Input: part model. Units: mm. Frame: model coordinates. Face numbers are marked on the shaded views. A direction names the side the tool comes from. Round coordinates to 2 decimals unless told otherwise and drop trailing zeros. Loops run counter-clockwise (first coordinate to the right, second up) from the corner with the lowest first, then second, coordinate; pieces in that order, holes last.
1) Access query for the marked faces 1 and 2. Directions: +Z, -Z, +X, -X, +Y, -Y. A direction counts if a zero-diameter tool reaches every point of the face in a straight line with its end or side. Return the directions, or none.
2) Section D-D, the plane z = -15. Return loops of the section in (x, y), and give its area (3 significant figures).
3) Section A-A, the plane y = 37. Return loops of the section in (x, z).
4) Section C-C, the plane x = -9.5. Return loops of the section in (y, z), and give its area (3 significant figures).
5) Draft query along Z for the marked faces 3, 4 and 5. Return one class per face: pulls with the +Z half, pulls with the -Z half, needs draft (parallel to the pull), parting line crosses it, or undercut.
6) Section B-B, the plane z = 0. Return loops of the section in (x, y).
7) Ray query, line 1 along X through (y, z) = (19.5, 0); line 2 along Y through (x, z) = (17, 0); line 3 along X through (y, z) = (35, 16). Return the intervals inside material, ascending.
8) First-contact query: pin 1 (3 mm diameter, centred on x = -5, y = 28.5, fed in from -Z); pin 2 (2 mm diameter, centred on x = 13, z = -18, fed in from -Y); pin 3 (5 mm diameter, centred on y = 9.5, z = 9.5, fed in from +X). Flat tips, straight axial feed; report the tip coordinate or a pass-through.
from build123d import *

# Parameters (mm, degrees)
SKETCH1_R           = 14
BOSS_EXTRUDE1_DEPTH = 32
BOSS_EXTRUDE2_DEPTH = 10
SKETCH6_R           = 8
CUT_EXTRUDE1_DEPTH  = 53.324865011
SKETCH8_R           = 2.75
CUT_EXTRUDE2_DEPTH  = 53.324865011
SKETCH9_R           = 2.75
CUT_EXTRUDE3_DEPTH  = 63.752621447


with BuildPart() as part:
    # Sketch1 → Boss-Extrude1 (new body)
    with BuildSketch(Plane(origin=(0, 0, 0), x_dir=(1, 0, 0), z_dir=(0, 1, 0))):
        with Locations(Location((0, 0, 0), (0, 0, 270))):
            Circle(SKETCH1_R)
    extrude(amount=BOSS_EXTRUDE1_DEPTH)

    # Sketch5 → Boss-Extrude2 (add)
    with BuildSketch(Plane(origin=(0, 32, 0), x_dir=(-1, 0, 0), z_dir=(0, 1, 0))):
        with BuildLine():
            Line((-20, 13.186792576), (-20, -13.186792576))
            ThreePointArc((-20, -13.186792576), (0, -23.956032611), (20, -13.186792576))
            Line((20, -13.186792576), (20, 13.186792576))
            ThreePointArc((20, 13.186792576), (0, 23.956032611), (-20, 13.186792576))
        make_face()
    extrude(amount=BOSS_EXTRUDE2_DEPTH)

    # Sketch6 → Cut-Extrude1 (cut, through all)
    with BuildSketch(Plane(origin=(0, 42, 0), x_dir=(-1, 0, 0), z_dir=(0, 1, 0))):
        with Locations(Location((0, 0, 0), (0, 0, 90))):
            Circle(SKETCH6_R)
    extrude(amount=-CUT_EXTRUDE1_DEPTH, mode=Mode.SUBTRACT)

    # Sketch8 → Cut-Extrude2 (cut, through all)
    with BuildSketch(Plane(origin=(0, 42, 0), x_dir=(-1, 0, 0), z_dir=(0, 1, 0))):
        with Locations(Location((0, 19, 0), (0, 0, 90))):
            Circle(SKETCH8_R)
        with Locations(Location((9.5, 16.454482672, 0), (0, 0, 90))):
            Circle(SKETCH8_R)
        with Locations(Location((9.5, -16.454482672, 0), (0, 0, 90))):
            Circle(SKETCH8_R)
        with Locations(Location((0, -19, 0), (0, 0, 90))):
            Circle(SKETCH8_R)
        with Locations(Location((-9.5, -16.454482672, 0), (0, 0, 90))):
            Circle(SKETCH8_R)
        with Locations(Location((-9.5, 16.454482672, 0), (0, 0, 90))):
            Circle(SKETCH8_R)
    extrude(amount=-CUT_EXTRUDE2_DEPTH, mode=Mode.SUBTRACT)

    # Sketch9 → Cut-Extrude3 (cut, through all)
    with BuildSketch(Plane(origin=(20, 0, 0), x_dir=(0, 0, -1), z_dir=(1, 0, 0))):
        with Locations((0, 37)):
            Circle(SKETCH9_R)
    extrude(amount=-CUT_EXTRUDE3_DEPTH, mode=Mode.SUBTRACT)


solid = part.part
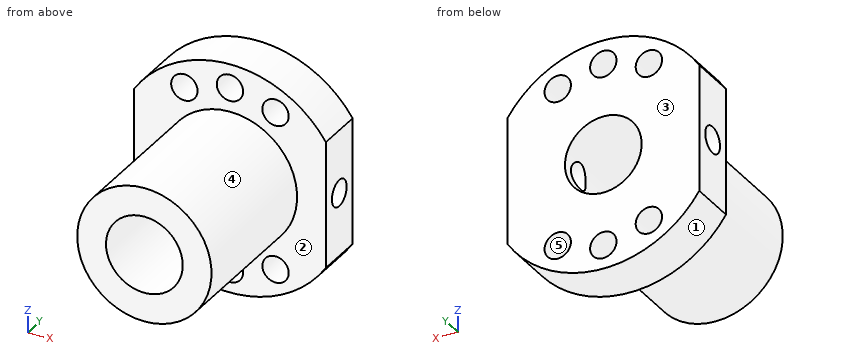
Final values:
1. face 1: -Z, +Y, -Y
1. face 2: -Y
2. outline: (-18.68, 32) - (-11.83, 32) - (-11.83, 42) - (-18.68, 42) - close; (-7.17, 32) - (7.17, 32) - (7.17, 42) - (-7.17, 42) - close; (11.83, 32) - (18.68, 32) - (18.68, 42) - (11.83, 42) - close
2. area: 280 mm2
3. outline: (-20, -13.19) arc R23.96 ccw to (20, -13.19) - (20, -2.75) - (7.51, -2.75) arc R8 cw to (-7.51, -2.75) - (-20, -2.75) - close; (-20, 2.75) - (-7.51, 2.75) arc R8 cw to (7.51, 2.75) - (20, 2.75) - (20, 13.19) arc R23.96 ccw to (-20, 13.19) - close; hole circle Ø5.5 at (-9.5, -16.45); hole circle Ø5.5 at (-9.5, 16.45); hole circle Ø5.5 at (0, -19); hole circle Ø5.5 at (0, 19); hole circle Ø5.5 at (9.5, -16.45); hole circle Ø5.5 at (9.5, 16.45)
4. outline: (0, -10.28) - (32, -10.28) - (32, -13.7) - (42, -13.7) - (42, 13.7) - (32, 13.7) - (32, 10.28) - (0, 10.28) - close; (32, -21.99) - (42, -21.99) - (42, -19.2) - (32, -19.2) - close; (32, 19.2) - (42, 19.2) - (42, 21.99) - (32, 21.99) - close; hole circle Ø5.5 at (37, 0)
4. area: 964 mm2
5. face 3: needs draft
5. face 4: parting line crosses it
5. face 5: undercut
6. outline: (-20, 32) - (-14, 32) - (-14, 0) - (-8, 0) - (-8, 34.25) - (-20, 34.25) - close; (-20, 39.75) - (-8, 39.75) - (-8, 42) - (-20, 42) - close; (8, 0) - (14, 0) - (14, 32) - (20, 32) - (20, 34.25) - (8, 34.25) - close; (8, 39.75) - (20, 39.75) - (20, 42) - (8, 42) - close
7. line 1: x = -14 to -8, 8 to 14
7. line 2: y = 32 to 34.25, 39.75 to 42
7. line 3: x = -17.83 to -12.21, -6.79 to 6.79, 12.21 to 17.83
8. pin 1: stops at z = -13.56
8. pin 2: stops at y = 32
8. pin 3: stops at x = 12.12
